```python
from build123d import *

# Parameters (mm, degrees)
SALIENTE_EXTRUIR1_DEPTH = 12
CROQUIS2_R              = 4.71
SALIENTE_EXTRUIR2_DEPTH = 30.5
CROQUIS3_R              = 2.425
SALIENTE_EXTRUIR3_DEPTH = 18


with BuildPart() as part:
    # Croquis1 → Saliente-Extruir1 (new body)
    with BuildSketch(Plane.XY):
        Polygon((0, 7.216878365), (-6.25, 3.608439182), (-6.25, -3.608439182), (0, -7.216878365), (6.25, -3.608439182), (6.25, 3.608439182), align=None)
    extrude(amount=SALIENTE_EXTRUIR1_DEPTH)

    # Croquis2 → Saliente-Extruir2 (add)
    with BuildSketch(Plane.XY.offset(12)):
        with Locations(Location((0, 0, 0), (0, 0, 180))):
            Circle(CROQUIS2_R)
    extrude(amount=SALIENTE_EXTRUIR2_DEPTH)

    # Croquis3 → Saliente-Extruir3 (add)
    with BuildSketch(Plane.XY.offset(42.5)):
        Circle(CROQUIS3_R)
    extrude(amount=SALIENTE_EXTRUIR3_DEPTH)


solid = part.part
```
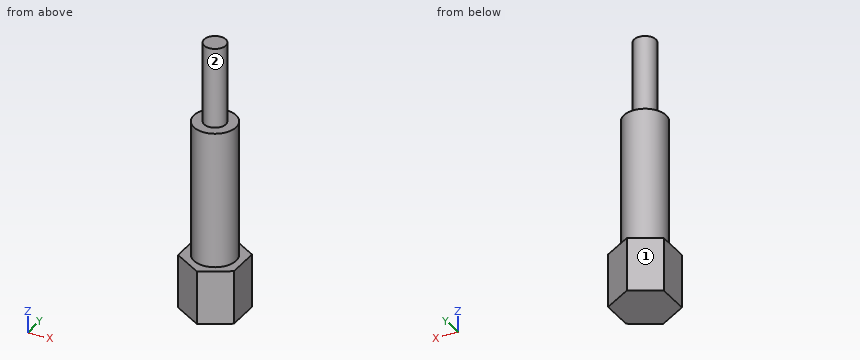
The model under review builds one solid part; all positions refer to its coordinate system, in mm. Face numbers are marked on the shaded views. A direction names the side the tool comes from. Round coordinates to 2 decimals unless told otherwise and drop trailing zeros. Loops run counter-clockwise (first coordinate to the right, second up) from the corner with the lowest first, then second, coordinate; pieces in that order, holes last.
Item 1: Take a section at D-D (z = 48.5). Write out the cut boundary in (x, y) (3 decimals), then the cut area to 3 significant figures.
Determined:
outline: circle Ø4.85 at (0, 0)
area: 18.5 mm2
Item 2: Take a section at C-C (z = 8.5). Write out the cut boundary in (x, y).
Determined:
outline: (-6.25, -3.61) - (0, -7.22) - (6.25, -3.61) - (6.25, 3.61) - (0, 7.22) - (-6.25, 3.61) - close
Item 3: Take a section at A-A (y = 0). Write out the cut boundary in (x, z) (3 decimals), then the cut area to 3 significant figures.
Determined:
outline: (-6.25, 0) - (6.25, 0) - (6.25, 12) - (4.71, 12) - (4.71, 42.5) - (2.425, 42.5) - (2.425, 60.5) - (-2.425, 60.5) - (-2.425, 42.5) - (-4.71, 42.5) - (-4.71, 12) - (-6.25, 12) - close
area: 525 mm2
Item 4: For the marked faces 1 and 2, list the 3-axis set-ups (+Z, -Z, +X, -X, +Y, -Y) from which the entire face can be reached by the end or side of a thin tool; tool diameter is ignored.
Determined:
face 1: +Z, -Z, -X, +Y
face 2: +Z
Item 5: Take a section at B-B (x = -3.5). Write out the cut boundary in (y, z), then the cut area to 3 significant figures.
Determined:
outline: (-5.2, 0) - (5.2, 0) - (5.2, 12) - (3.15, 12) - (3.15, 42.5) - (-3.15, 42.5) - (-3.15, 12) - (-5.2, 12) - close
area: 317 mm2
Item 6: For line 1 (Y direction, x = 0, z = 38); line 2 (Z direction, x = 2.25, y = -4.75); line 3 (Z direction, x = 0, y = -3.5), list the stretches that pass through material, from the lowest coordinate up.
Determined:
line 1: y = -4.71 to 4.71
line 2: z = 0 to 12
line 3: z = 0 to 42.5
Item 7: Clearance check with flat-ended pins moving along their axes: pin 1 Ø4 at (x, z) = (-1, 24) entering from -Y; pin 2 Ø2 at (x, z) = (4.5, 20) entering from +Y. State where each tip first meets the part, or that it passes through.
Determined:
pin 1: stops at y = -4.71
pin 2: stops at y = 3.15
